Build history of the part. All positions in model axes, mm. Give positions to 0.01 mm unless a question says otherwise; leave off trailing zeros. Write each loop counter-clockwise with the first axis right and the second up, starting at its lowest first coordinate (ties: lowest second). Pieces come first, ordered by that corner, then holes. Notation, with made-up numbers: (31.5, 89) -> (43.5, 89) arc R14 cw to (43.5, 114) -> close; hole circle Ø8 at (-28.75, 69.5). An arc over 180 degrees is marked (long way). Put each result on its own line as item: value. Start each with the question number.
Item 1: Drill centre lines: line 1 along Z through (x, y) = (0, -1); line 2 along X through (y, z) = (-1.15, 0.25); line 3 along X through (y, z) = (-1.1, 0.75). Where is each one in solid material? Low to high.
Item 2: Slice it at B-B, the plane y = -0.5. List the corners of the cut face in (x, z).
Item 3: Slice it at A-A, the plane z = 0. List the corners of the cut face in (x, y).
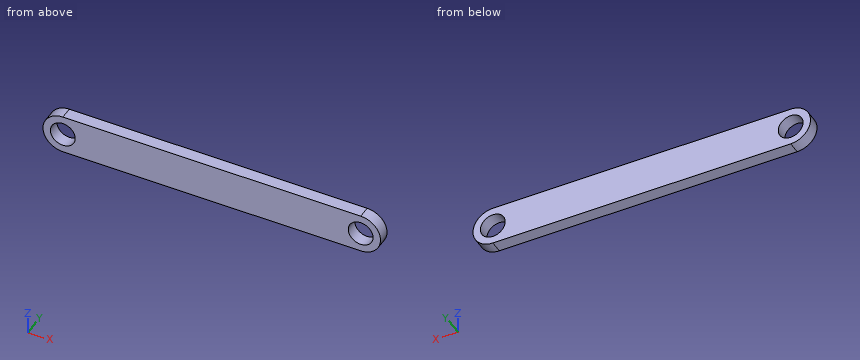
```python
from build123d import *

# Parameters (mm, degrees)
F0_R     = 2.5
F1_DEPTH = 2.5


with BuildPart() as f1:
    # F0 (on Front) → F1 (new body)
    with BuildSketch(Plane.XZ):
        with BuildLine():
            Line((60, 4), (0, 4))
            ThreePointArc((0, 4), (-4, 0), (0, -4))
            Line((0, -4), (60, -4))
            ThreePointArc((60, -4), (64, 0), (60, 4))
        make_face()
        Circle(F0_R, mode=Mode.SUBTRACT)
        with BuildLine():
            ThreePointArc((57.5, 0), (60, 2.5), (62.5, 0))
            ThreePointArc((62.5, 0), (60, -2.5), (57.5, 0))
        make_face(mode=Mode.SUBTRACT)
    extrude(amount=F1_DEPTH)


solid = f1.part
```
Values follow:
1. line 1: -4 to -2.5, 2.5 to 4
1. line 2: -3.99 to -2.49, 2.49 to 57.51, 62.49 to 63.99
1. line 3: -3.93 to -2.38, 2.38 to 57.62, 62.38 to 63.93
2. outline: (0, -4) -> (60, -4) arc R4 ccw to (60, 4) -> (0, 4) arc R4 ccw to start; hole circle Ø5 at (0, 0); hole circle Ø5 at (60, 0)
3. outline: (-4, -2.5) -> (-2.5, -2.5) -> (-2.5, 0) -> (-4, 0) -> close; (2.5, -2.5) -> (57.5, -2.5) -> (57.5, 0) -> (2.5, 0) -> close; (62.5, -2.5) -> (64, -2.5) -> (64, 0) -> (62.5, 0) -> close
